CAD build for the part. Positions are in the model's coordinates, mm. A direction names the side the tool comes from. Give positions to 0.01 mm unless a question says otherwise; leave off trailing zeros. Write each loop counter-clockwise with the first axis right and the second up, starting at its lowest first coordinate (ties: lowest second). Pieces come first, ordered by that corner, then holes. Notation, with made-up numbers: (13, 48) -> (22, 48) arc R32 cw to (22, 77) -> close; hole circle Ø4 at (-1, 13). An arc over 180 degrees is marked (long way). Answer as a JSON object with one key per item and string values.
```python
from build123d import *

# Parameters (mm, degrees)
SKETCH1_R               = 7.9375
SKETCH1_R_2             = 11.1125
BOSS_EXTRUDE1_DEPTH     = 12.7
F_8_CLEARANCE_HOLE1_D   = 4.4958
SKETCH5_R               = 18.415
CUT_EXTRUDE1_DEPTH      = 13.7
SKETCH7_R               = 9.525
CUT_EXTRUDE2_DEPTH      = 13.7
CUT_EXTRUDE3_DEPTH      = 13.7
BOSS_EXTRUDE2_DEPTH     = 12.7
CUT_EXTRUDE4_DEPTH      = 13.7
SKETCH11_W              = 12.7
SKETCH11_H              = 178.054
CUT_EXTRUDE5_DEPTH      = 3.175
BOSS_EXTRUDE3_DEPTH     = 19.05
CUT_EXTRUDE6_DEPTH      = 20.05
F_3_8_CLEARANCE_HOLE1_D = 10.0838
CUT_EXTRUDE7_DEPTH      = 20.05
BOSS_EXTRUDE4_DEPTH     = 19.05
FILLET1_R               = 19.05
FILLET2_R               = 9.525
CUT_EXTRUDE8_DEPTH      = 20.05
BOSS_EXTRUDE5_DEPTH     = 19.05
FILLET3_R               = 4.7625


with BuildPart() as part:
    # Sketch1 → Boss-Extrude1 (new body)
    with BuildSketch(Plane(origin=(0, 0, 0), x_dir=(0, 0, -1), z_dir=(1, 0, 0))):
        with BuildLine():
            Line((93.345, 0), (55.245, 50.8))
            Line((55.245, 50.8), (-160.655, 50.8))
            ThreePointArc((-160.655, 50.8), (-211.455, 0), (-160.655, -50.8))
            Line((-160.655, -50.8), (55.245, -50.8))
            Line((55.245, -50.8), (93.345, 0))
        make_face()
        with Locations((-88.9, 0)):
            Circle(SKETCH1_R, mode=Mode.SUBTRACT)
        with Locations((-38.1, 0)):
            Circle(SKETCH1_R, mode=Mode.SUBTRACT)
        with Locations((-160.655, 0)):
            Circle(SKETCH1_R_2, mode=Mode.SUBTRACT)
        Circle(SKETCH1_R, mode=Mode.SUBTRACT)
    extrude(amount=BOSS_EXTRUDE1_DEPTH)

    # #8 Clearance Hole1 (through all)
    with Locations(Plane.ZY):
        with Locations((-17.691104559, 17.691104559), (17.691104559, 17.691104559), (17.691104559, -17.691104559), (-17.691104559, -17.691104559)):
            Hole(F_8_CLEARANCE_HOLE1_D / 2)

    # Sketch5 → Cut-Extrude1 (cut, through all)
    with BuildSketch(Plane.ZY):
        Circle(SKETCH5_R)
    extrude(amount=-CUT_EXTRUDE1_DEPTH, mode=Mode.SUBTRACT)

    # Sketch7 → Cut-Extrude2 (cut, through all)
    with BuildSketch(Plane.ZY):
        with Locations((-55.245, 0)):
            Circle(SKETCH7_R)
    extrude(amount=-CUT_EXTRUDE2_DEPTH, mode=Mode.SUBTRACT)

    # Sketch8 → Cut-Extrude3 (cut, through all)
    with BuildSketch(Plane(origin=(12.7, 0, 0), x_dir=(0, 0, -1), z_dir=(1, 0, 0))):
        Polygon((-160.655, 50.8), (-211.455, 25.4), (-211.455, -25.4), (-160.655, -50.8), (-233.239745749, -50.8), (-233.239745749, 50.8), align=None)
    extrude(amount=-CUT_EXTRUDE3_DEPTH, mode=Mode.SUBTRACT)

    # Sketch9 → Boss-Extrude2 (add)
    with BuildSketch(Plane(origin=(12.7, 0, 0), x_dir=(0, 0, -1), z_dir=(1, 0, 0))):
        Polygon((-160.655, 50.8), (-211.455, 25.4), (-211.455, 0), (-211.455, -25.4), (-160.655, -50.8), (-160.655, -40.64), (-202.749323348, 0), (-160.655, 40.64), align=None)
    extrude(amount=-BOSS_EXTRUDE2_DEPTH)

    # Sketch10 → Cut-Extrude4 (cut, through all)
    with BuildSketch(Plane.ZY):
        Polygon((-79.0575, -19.05), (-79.0575, 19.05), (-93.345, 0), align=None)
    extrude(amount=-CUT_EXTRUDE4_DEPTH, mode=Mode.SUBTRACT)

    # Sketch11 → Cut-Extrude5 (cut)
    with BuildSketch(Plane(origin=(0, 50.8, 0), x_dir=(1, 0, 0), z_dir=(0, 1, 0))):
        with Locations((6.35, -52.705)):
            Rectangle(SKETCH11_W, SKETCH11_H)
    cut_extrude5 = extrude(amount=-CUT_EXTRUDE5_DEPTH, mode=Mode.SUBTRACT)

    # Mirror1: Cut-Extrude5 across plane
    add(cut_extrude5.mirror(Plane.ZX), mode=Mode.SUBTRACT)

    # Sketch13 → Cut-Extrude6 (cut, through all)
    with BuildSketch(Plane(origin=(12.7, 0, 0), x_dir=(0, 0, -1), z_dir=(1, 0, 0))):
        Polygon((-161.254612663, -53.34), (-139.192, -53.34), (-139.192, -50.165), (33.782, -50.165), (33.782, -53.34), (56.515, -53.34), (81.5975, -19.896666667), (81.5975, 19.896666667), (56.515, 53.34), (33.782, 53.34), (33.782, 50.165), (-139.192, 50.165), (-139.192, 53.34), (-161.254612663, 53.34), (-213.995, 26.969806331), (-213.995, -26.969806331), align=None)
    extrude(amount=-CUT_EXTRUDE6_DEPTH, mode=Mode.SUBTRACT)


with BuildPart() as body_2:
    # Sketch12 → Boss-Extrude3 (new body)
    with BuildSketch(Plane(origin=(12.7, 0, 0), x_dir=(0, 0, -1), z_dir=(1, 0, 0))):
        with BuildLine():
            ThreePointArc((-211.89681554, -56.397839854), (-236.855, 0), (-211.89681554, 56.397839854))
            Line((-211.89681554, 56.397839854), (-243.205, 43.989212666))
            Line((-243.205, 43.989212666), (-243.205, -43.989212666))
            Line((-243.205, -43.989212666), (-211.89681554, -56.397839854))
        make_face()
        with BuildLine():
            Line((-217.805, 29.324515829), (-162.154031657, 57.15))
            Line((-162.154031657, 57.15), (-166.916531657, 66.675))
            Line((-166.916531657, 66.675), (-185.966531657, 66.675))
            Line((-185.966531657, 66.675), (-211.89681554, 56.397839854))
            ThreePointArc((-211.89681554, 56.397839854), (-236.855, 0), (-211.89681554, -56.397839854))
            Line((-211.89681554, -56.397839854), (-185.966531657, -66.675))
            Line((-185.966531657, -66.675), (-166.916531657, -66.675))
            Line((-166.916531657, -66.675), (-162.154031657, -57.15))
            Line((-162.154031657, -57.15), (-217.805, -29.324515829))
            Line((-217.805, -29.324515829), (-217.805, 29.324515829))
        make_face()
    extrude(amount=-BOSS_EXTRUDE3_DEPTH)

    # 3/8 Clearance Hole1 (through all)
    with Locations(Plane(origin=(12.7, 0, 0), x_dir=(0, 0, -1), z_dir=(1, 0, 0))):
        with Locations((-230.505, 0), (-230.505, 33.690140829), (-202.106936686, 47.889172486), (-230.505, -33.690140829), (-202.106936686, -47.889172486)):
            Hole(F_3_8_CLEARANCE_HOLE1_D / 2)

    # Sketch16 → Cut-Extrude7 (cut, through all)
    with BuildSketch(Plane(origin=(12.7, 0, 0), x_dir=(0, 0, -1), z_dir=(1, 0, 0))):
        with BuildLine():
            ThreePointArc((-190.589767426, 47.889172486), (-190.722432786, 46.146112328), (-191.117372542, 44.443208515))
            Line((-191.117372542, 44.443208515), (-162.86398324, 58.569903166))
            Line((-162.86398324, 58.569903166), (-166.916531657, 66.675))
            Line((-166.916531657, 66.675), (-185.966531657, 66.675))
            Line((-185.966531657, 66.675), (-206.35048523, 58.596062021))
            ThreePointArc((-206.35048523, 58.596062021), (-195.635015761, 57.415946719), (-190.589767426, 47.889172486))
        make_face()
        with BuildLine():
            Line((-162.86398324, 58.569903166), (-191.117372542, 44.443208515))
            ThreePointArc((-191.117372542, 44.443208515), (-191.551739911, 43.281243579), (-192.108559765, 42.172735946))
            Line((-192.108559765, 42.172735946), (-162.154031657, 57.15))
            Line((-162.154031657, 57.15), (-162.86398324, 58.569903166))
        make_face()
        with BuildLine():
            Line((-191.117372542, 44.443208515), (-205.943903995, 37.029942788))
            ThreePointArc((-205.943903995, 37.029942788), (-204.753711625, 36.680257722), (-203.532813606, 36.460609025))
            Line((-203.532813606, 36.460609025), (-192.108559765, 42.172735946))
            ThreePointArc((-192.108559765, 42.172735946), (-191.551739911, 43.281243579), (-191.117372542, 44.443208515))
        make_face()
        with BuildLine():
            Line((-219.3925, 30.305644786), (-219.3925, -30.305644786))
            Line((-219.3925, -30.305644786), (-205.943903995, -37.029942788))
            ThreePointArc((-205.943903995, -37.029942788), (-204.753711625, -36.680257722), (-203.532813606, -36.460609025))
            Line((-203.532813606, -36.460609025), (-217.805, -29.324515829))
            Line((-217.805, -29.324515829), (-217.805, 29.324515829))
            Line((-217.805, 29.324515829), (-203.532813606, 36.460609025))
            ThreePointArc((-203.532813606, 36.460609025), (-204.753711625, 36.680257722), (-205.943903995, 37.029942788))
            Line((-205.943903995, 37.029942788), (-219.3925, 30.305644786))
        make_face()
        with BuildLine():
            ThreePointArc((-203.532813606, -36.460609025), (-204.753711625, -36.680257722), (-205.943903995, -37.029942788))
            Line((-205.943903995, -37.029942788), (-191.117372542, -44.443208515))
            ThreePointArc((-191.117372542, -44.443208515), (-191.551739911, -43.281243579), (-192.108559765, -42.172735946))
            Line((-192.108559765, -42.172735946), (-203.532813606, -36.460609025))
        make_face()
        with BuildLine():
            ThreePointArc((-192.108559765, -42.172735946), (-191.551739911, -43.281243579), (-191.117372542, -44.443208515))
            Line((-191.117372542, -44.443208515), (-162.86398324, -58.569903166))
            Line((-162.86398324, -58.569903166), (-162.154031657, -57.15))
            Line((-162.154031657, -57.15), (-192.108559765, -42.172735946))
        make_face()
        with BuildLine():
            Line((-162.86398324, -58.569903166), (-191.117372542, -44.443208515))
            ThreePointArc((-191.117372542, -44.443208515), (-190.722432786, -46.146112328), (-190.589767426, -47.889172486))
            Line((-190.589767426, -47.889172486), (-190.589767426, -64.842635395))
            Line((-190.589767426, -64.842635395), (-185.966531657, -66.675))
            Line((-185.966531657, -66.675), (-166.916531657, -66.675))
            Line((-166.916531657, -66.675), (-162.86398324, -58.569903166))
        make_face()
    extrude(amount=-CUT_EXTRUDE7_DEPTH, mode=Mode.SUBTRACT)

    # Sketch17 → Boss-Extrude4 (add)
    with BuildSketch(Plane(origin=(12.7, 0, 0), x_dir=(0, 0, -1), z_dir=(1, 0, 0))):
        Polygon((-338.455, -73.025), (-211.234676528, -73.025), (-190.589767426, -64.842635395), (-243.205, -43.989212666), (-243.205, 43.989212666), (-255.905, 38.955718453), (-287.655, -57.15), (-351.768316876, -66.675), (-361.293316876, -76.2), (-344.805, -76.2), align=None)
    extrude(amount=-BOSS_EXTRUDE4_DEPTH)

    # Fillet1
    fillet1_edges = [body_2.edges().sort_by_distance(p)[0] for p in [
        (3.175, -73.025, 211.234676528),
        (3.175, -57.15, 287.655),
        (3.175, 38.955718453, 255.905),
        (3.175, -64.842635395, 190.589767426),
    ]]
    fillet(fillet1_edges, radius=FILLET1_R)

    # Fillet2
    fillet2_edges = [body_2.edges().sort_by_distance(p)[0] for p in [
        (3.175, -73.025, 338.455),
        (3.175, -76.2, 344.805),
        (3.175, -66.675, 351.768316876),
    ]]
    fillet(fillet2_edges, radius=FILLET2_R)

    # Sketch18 → Cut-Extrude8 (cut, through all)
    with BuildSketch(Plane(origin=(12.7, 0, 0), x_dir=(0, 0, -1), z_dir=(1, 0, 0))):
        with BuildLine():
            ThreePointArc((-273.120706312, -49.592608078), (-276.117108341, -56.027596012), (-280.520687302, -61.595))
            Line((-280.520687302, -61.595), (-214.872157895, -61.595))
            ThreePointArc((-214.872157895, -61.595), (-213.442985613, -61.459775654), (-212.064537448, -61.058901992))
            Line((-212.064537448, -61.058901992), (-206.832146979, -58.985106153))
            ThreePointArc((-206.832146979, -58.985106153), (-206.472989442, -58.831999008), (-206.122145618, -58.660696511))
            Line((-206.122145618, -58.660696511), (-207.218588082, -58.112475279))
            Line((-207.218588082, -58.112475279), (-241.935, -40.75426932))
            Line((-241.935, -40.75426932), (-241.935, 32.197558556))
            Line((-241.935, 32.197558556), (-243.416943097, 31.610208005))
            ThreePointArc((-243.416943097, 31.610208005), (-246.152147631, 29.755215195), (-247.844705879, 26.916625978))
            Line((-247.844705879, 26.916625978), (-273.120706312, -49.592608078))
        make_face()
    extrude(amount=-CUT_EXTRUDE8_DEPTH, mode=Mode.SUBTRACT)

    # Sketch19 → Boss-Extrude5 (add)
    with BuildSketch(Plane(origin=(12.7, 0, 0), x_dir=(0, 0, -1), z_dir=(1, 0, 0))):
        with BuildLine():
            ThreePointArc((-243.416943097, 31.610208005), (-246.152147631, 29.755215195), (-247.844705879, 26.916625978))
            Line((-247.844705879, 26.916625978), (-251.219614601, 16.700940075))
            ThreePointArc((-251.219614601, 16.700940075), (-245.940917069, 19.909009969), (-241.935, 15.206990348))
            Line((-241.935, 15.206990348), (-241.935, 32.197558556))
            Line((-241.935, 32.197558556), (-243.416943097, 31.610208005))
        make_face()
        with BuildLine():
            ThreePointArc((-271.08233553, -61.595), (-275.17466524, -59.268530337), (-275.268808735, -54.562070888))
            ThreePointArc((-275.268808735, -54.562070888), (-277.640258261, -58.268577072), (-280.520687302, -61.595))
            Line((-280.520687302, -61.595), (-271.08233553, -61.595))
        make_face()
        with BuildLine():
            Line((-206.122145618, -58.660696511), (-218.297957405, -52.572790618))
            ThreePointArc((-218.297957405, -52.572790618), (-216.376587841, -54.328705688), (-215.665312383, -56.8325))
            ThreePointArc((-215.665312383, -56.8325), (-217.060216337, -60.200096045), (-220.427812383, -61.595))
            Line((-220.427812383, -61.595), (-214.872157895, -61.595))
            ThreePointArc((-214.872157895, -61.595), (-213.442985613, -61.459775654), (-212.064537448, -61.058901992))
            Line((-212.064537448, -61.058901992), (-206.832146979, -58.985106153))
            ThreePointArc((-206.832146979, -58.985106153), (-206.472989442, -58.831999008), (-206.122145618, -58.660696511))
        make_face()
    extrude(amount=-BOSS_EXTRUDE5_DEPTH)

    # Fillet3
    fillet3_edges = [body_2.edges().sort_by_distance(p)[0] for p in [
        (3.175, -40.75426932, 241.935),
    ]]
    fillet(fillet3_edges, radius=FILLET3_R)


solid = body_2.part
```
1) Wall check: probe 1 along Z at (x, y) = (11.25, 1) (1 decimal); probe 2 along Y at (x, z) = (11.75, 228) (3 decimals); probe 3 along Z at (x, y) = (2.5, -44). Give the ranges that are in metal, low to high.
Model answer:
{"probe 1": "z = 219.4 to 225.6, 235.4 to 241.9, 256.4 to 268.4", "probe 2": "y = -73.025 to -61.595, -47.722 to -38.066, -29.315 to -4.376, 4.376 to 29.315, 38.066 to 50.016", "probe 3": "z = 192 to 198.9, 205.32 to 235.44, 271.27 to 283.31"}
2) Pin check, flat tips, straight feed: pin 1 (6 mm diameter, centred on x = -2, z = 284.5, fed in from -Y) (3 decimals); pin 2 (1.5 mm diameter, centred on x = 10.5, y = 14, fed in from +Z); pin 3 (3 mm diameter, centred on x = 10, y = -11, fed in from -Z). Stop position of each tip, or through.
Model answer:
{"pin 1": "stops at y = -73.025", "pin 2": "stops at z = 264.4", "pin 3": "stops at z = 219.39"}
3) Slice it at C-C (y = 0). State how many separate pieces and enclosed holes the cut face has, then the cut area to 3 significant figures.
Model answer:
{"separate pieces": "3", "enclosed holes": "0", "area": "467 mm2"}
4) 3-axis set-ups, long thin cutter, end or side, ignore diameter. For faces 5 (the flat face through (3.31, -7.22, 271.16)), 6 (the flat face through (3, 0, 219.392)), 7 (the cylindrical face through (3.308, -59.328, 275.139)), 8 (the flat face through (3, -73.025, 276)): which of +Z, -Z, +X, -X, +Y, -Y reach the whole face in a straight line?
Model answer:
{"face 5": "+Z, +X, -X, +Y", "face 6": "-Z, +X, -X", "face 7": "+X, -X", "face 8": "-Z, +X, -X, -Y"}
5) Mould opens along Y. For faces 1 (the cylindrical face through (3.04, 37.68, 254.39)), 2 (the cylindrical face through (3.042, -62.737, 193.972)), 3 (the flat face through (-6.35, -23, 238)), 4 (the cylindrical face through (3.04, 48.11, 197.07)) say: released by +Y, released by -Y, zero draft, split by the parting line, or undercut.
Model answer:
{"face 1": "released by +Y", "face 2": "released by -Y", "face 3": "zero draft", "face 4": "undercut"}
6) Slice it at B-B (z = 268). List the corners of the cut face in (x, y) (3 decimals).
Model answer:
{"outline": "(-6.35, -73.025) -> (12.7, -73.025) -> (12.7, -61.595) -> (-6.35, -61.595) -> close; (-6.35, -34.092) -> (12.7, -34.092) -> (12.7, 2.345) -> (-6.35, 2.345) -> close"}
